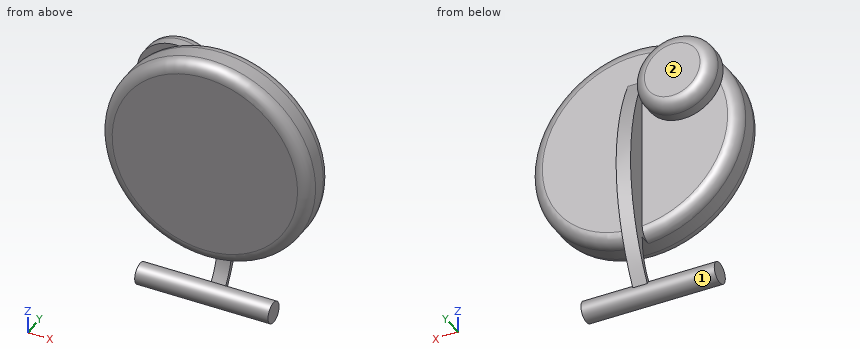
from build123d import *

# Parameters (mm, degrees)
SKETCH1_R           = 2.2606
BOSS_EXTRUDE1_DEPTH = 28.575
BOSS_EXTRUDE2_DEPTH = 3.0988
SKETCH3_R           = 22.4028
BOSS_EXTRUDE3_DEPTH = 8.255
FILLET1_R           = 2.54
SKETCH4_R           = 8.4963
BOSS_EXTRUDE4_DEPTH = 4.5974
FILLET2_R           = 2.54


with BuildPart() as part:
    # Sketch1 → Boss-Extrude1 (new body)
    with BuildSketch(Plane(origin=(0, 0, 0), x_dir=(0, 0, -1), z_dir=(1, 0, 0))):
        Circle(SKETCH1_R)
    extrude(amount=BOSS_EXTRUDE1_DEPTH)

    # Sketch2 → Boss-Extrude2 (add)
    with BuildSketch(Plane(origin=(17.5514, 0, 0), x_dir=(0, 0, -1), z_dir=(1, 0, 0))):
        with BuildLine():
            Line((-46.101, 4.1402), (-10.3124, 4.1402))
            ThreePointArc((-10.3124, 4.1402), (-4.725931778, 3.141811032), (0, 0))
            Line((0, 0), (2.2606, 0))
            ThreePointArc((2.2606, 0), (-21.350803051, 8.721215285), (-46.101, 4.1402))
        make_face()
    extrude(amount=-BOSS_EXTRUDE2_DEPTH)

    # Sketch3 → Boss-Extrude3 (add)
    with BuildSketch(Plane.XZ.offset(-4.1402)):
        with Locations(Location((16.002, 32.7152, 0), (0, 0, 270))):
            Circle(SKETCH3_R)
    extrude(amount=BOSS_EXTRUDE3_DEPTH)

    # Fillet1
    fillet1_edges = [part.edges().sort_by_distance(p)[0] for p in [
        (16.002, 4.1402, 55.118),
        (16.002, -4.1148, 55.118),
    ]]
    fillet(fillet1_edges, radius=FILLET1_R)

    # Sketch4 → Boss-Extrude4 (add)
    with BuildSketch(Plane(origin=(0, 4.1402, 0), x_dir=(1, 0, 0), z_dir=(0, 1, 0))):
        with Locations(Location((5.61488389, -43.318674516, 0), (0, 0, 159.448311982))):
            Circle(SKETCH4_R)
    extrude(amount=BOSS_EXTRUDE4_DEPTH)

    # Fillet2
    fillet2_edges = [part.edges().sort_by_distance(p)[0] for p in [
        (13.570444327, 8.7376, 46.301319621),
    ]]
    fillet(fillet2_edges, radius=FILLET2_R)


solid = part.part
Could you check a few things on this model? Use its own coordinates, in mm. Face numbers are marked on the shaded views. Coordinates: 2 decimals unless noted, no trailing zeros. Order: outer loops, then holes, each group sorted by start corner. A loop starts at its lowest first (then second) coordinate and runs counter-clockwise, first axis right, second up. Notation, with made-up numbers: (71.5, -6.5) - (85.5, -6.5) arc R36 ccw to (85.5, 29.5) - close; hole circle Ø1 at (-38.75, 54). An arc over 180 degrees is marked (long way). Answer in a Markdown table with one row per item. Add a question column.
(1) Will these pins go through, and if not, where does the flat tip stop? pin 1 (20 mm diameter, centred on x = 19, z = 42.5, fed in from +Y); pin 2 (2 mm diameter, centred on y = 6, z = 12.5, fed in from +X); pin 3 (3.5 mm diameter, centred on y = -0.5, z = 0, fed in from -X); pin 4 (3 mm diameter, centred on x = 24, y = 6.5, fed in from -Z).
(2) If we section it at C-C, the plane y = 0: Please give me the cut outline in (x, z) (3 decimals), then the cut area to 3 significant figures.
(3) I need wall thicknesses on L1, parallel to X at y = 5.5, z = 33.5; L2, parallel to Y at x = 2, z = 35; L3, parallel to Z at x = 6.5, y = -0.75. Which ranges of each line are inside material? Lowest first, please.
(4) If we section it at B-B, the plane z = 0: Please give me the cut outline in (x, y) (3 decimals), then the cut area to 3 significant figures.
(5) If we mould it in two halves opening along Z, with no side actions, what happens to the marked faces 1 and 2? For each: released by +Z, released by -Z, zero draft, split by the parting line, or undercut.
(6) If we section it at A-A, the plane y = 4.75: Please give me the cut outline in (x, z).
Results are:
| question | item | result |
|---|---|---|
| 1 | pin 1 | stops at y = 8.74 |
| 1 | pin 2 | stops at x = 17.55 |
| 1 | pin 3 | stops at x = 0 |
| 1 | pin 4 | passes through |
| 2 | outline | circle Ø44.806 at (16.002, 32.715); (0, -2.261) - (28.575, -2.261) - (28.575, 2.261) - (0, 2.261) - close |
| 2 | area | 1,710 mm2 |
| 3 | L1 | x = 14.45 to 17.55 |
| 3 | L2 | y = -4.11 to 4.14 |
| 3 | L3 | z = -2.13 to 2.13, 12.43 to 53 |
| 4 | outline | (0, -2.261) - (28.575, -2.261) - (28.575, 2.261) - (0, 2.261) - close |
| 4 | area | 129 mm2 |
| 5 | face 1 | undercut |
| 5 | face 2 | zero draft |
| 6 | outline | circle Ø16.99 at (5.61, 43.32); (14.45, 6) - (17.55, 6) - (17.55, 44.79) - (14.45, 44.79) - close |
